Input: part model. Units: mm. Frame: model coordinates. A direction names the side the tool comes from. Give positions to 0.01 mm unless a question says otherwise; leave off trailing zeros. Loops run counter-clockwise (first coordinate to the right, second up) from the corner with the lowest first, then second, coordinate; pieces in that order, holes last. Notation, with made-up numbers: (55.25, -39.75) - (71.25, -39.75) arc R12 cw to (71.25, -19.75) - close; hole circle Ø8 at (-28.75, 45). An arc over 180 degrees is marked (long way). Answer as a JSON object with one key per item and string values.
from build123d import *

# Parameters (mm, degrees)
SKETCH1_R           = 2.54
SKETCH1_W           = 20.32
SKETCH1_H           = 25.4
BOSS_EXTRUDE1_DEPTH = 3.175


with BuildPart() as part:
    # Sketch1 → Boss-Extrude1 (new body)
    with BuildSketch(Plane(origin=(0, 0, 0), x_dir=(1, 0, 0), z_dir=(0, 1, 0))):
        with BuildLine():
            Line((-28.4999938, 15.7999938), (-28.4999938, 9.525))
            Line((-28.4999938, 9.525), (-36.1199938, 9.525))
            ThreePointArc((-36.1199938, 9.525), (-39.712096248, 8.037102448), (-41.1999938, 4.445))
            Line((-41.1999938, 4.445), (-41.1999938, -4.445))
            ThreePointArc((-41.1999938, -4.445), (-39.712096248, -8.037102448), (-36.1199938, -9.525))
            Line((-36.1199938, -9.525), (-28.4999938, -9.525))
            Line((-28.4999938, -9.525), (-28.4999938, -15.7999938))
            Line((-28.4999938, -15.7999938), (-15.7999938, -15.7999938))
            Line((-15.7999938, -15.7999938), (-15.7999938, -28.4999938))
            Line((-15.7999938, -28.4999938), (15.7999938, -28.4999938))
            Line((15.7999938, -28.4999938), (15.7999938, -15.7999938))
            Line((15.7999938, -15.7999938), (28.4999938, -15.7999938))
            Line((28.4999938, -15.7999938), (28.4999938, -9.525))
            Line((28.4999938, -9.525), (36.1199938, -9.525))
            ThreePointArc((36.1199938, -9.525), (39.712096248, -8.037102448), (41.1999938, -4.445))
            Line((41.1999938, -4.445), (41.1999938, 4.445))
            ThreePointArc((41.1999938, 4.445), (39.712096248, 8.037102448), (36.1199938, 9.525))
            Line((36.1199938, 9.525), (28.4999938, 9.525))
            Line((28.4999938, 9.525), (28.4999938, 15.7999938))
            Line((28.4999938, 15.7999938), (15.7999938, 15.7999938))
            Line((15.7999938, 15.7999938), (15.7999938, 28.4999938))
            Line((15.7999938, 28.4999938), (-15.7999938, 28.4999938))
            Line((-15.7999938, 28.4999938), (-15.7999938, 15.7999938))
            Line((-15.7999938, 15.7999938), (-28.4999938, 15.7999938))
        make_face()
        with Locations((-34.8499938, 0)):
            Circle(SKETCH1_R, mode=Mode.SUBTRACT)
        with Locations((34.8499938, 0)):
            Circle(SKETCH1_R, mode=Mode.SUBTRACT)
        Rectangle(SKETCH1_W, SKETCH1_H, mode=Mode.SUBTRACT)
    extrude(amount=BOSS_EXTRUDE1_DEPTH)


solid = part.part
Item 1: Cut plane B-B (y = 2.2). Give the number of separate pieces and of enclosed holes in the cut face, then the cut area to 3 significant figures.
Geometry check:
{"separate pieces": "1", "enclosed holes": "3", "area": "2,510 mm2"}
Item 2: Mould query, pull axis X, two halves, no side actions, for faces 5 (the face through (-28.5, 2, 13)), 6 (the face through (32.312, 1.565, -0.112)), 7 (the face through (0, 2, 28.5)), 8 (the face through (39.67, 1.57, 8.08)). Classes: released by +X, released by -X, zero draft, split by the parting line, or undercut.
Geometry check:
{"face 5": "released by -X", "face 6": "undercut", "face 7": "zero draft", "face 8": "released by +X"}
Item 3: Cut plane C-C (x = -20). Return loops of the section in (y, z) (3 decimals).
Geometry check:
{"outline": "(0, -15.8) - (3.175, -15.8) - (3.175, 15.8) - (0, 15.8) - close"}
Item 4: Contact query for flat-ended pins moving along their axis: P1, Ø1, axis at x = -30.5, y = 1, coming from the +Z side (3 decimals); P2, Ø1, axis at x = -21, y = 1, coming from the -Z side; P3, Ø1, axis at x = -21, y = 1.5, coming from the +Z side; P4, Ø4.5, axis at x = 34.85, z = 0, coming from the +Y side. Output: stop coordinate, or through.
Geometry check:
{"P1": "stops at z = 9.525", "P2": "stops at z = -15.8", "P3": "stops at z = 15.8", "P4": "passes through"}
Item 5: Access query for faces 1 (the face through (0, 2, 12.7)), 2 (the face through (28.5, 2, -13)), 3 (the face through (28.5, 2, 13)), 4 (the face through (-15.8, 2, -22)). Directions: +Z, -Z, +X, -X, +Y, -Y. A direction counts if a zero-diameter tool reaches every point of the face in a straight line with its end or side. Return the directions, or none.
Geometry check:
{"face 1": "+Y, -Y", "face 2": "-Z, +X, +Y, -Y", "face 3": "+Z, +X, +Y, -Y", "face 4": "-Z, -X, +Y, -Y"}
Item 6: Cut plane A-A (z = 0). Return loops of the section in (x, y) (3 decimals).
Geometry check:
{"outline": "(-41.2, 0) - (-37.39, 0) - (-37.39, 3.175) - (-41.2, 3.175) - close; (-32.31, 0) - (-10.16, 0) - (-10.16, 3.175) - (-32.31, 3.175) - close; (10.16, 0) - (32.31, 0) - (32.31, 3.175) - (10.16, 3.175) - close; (37.39, 0) - (41.2, 0) - (41.2, 3.175) - (37.39, 3.175) - close"}
Item 7: Material intervals for line 1 (X direction, y = 2.25, z = 0); line 2 (Z direction, x = 0, y = 2.3); line 3 (Z direction, x = 35, y = 2.05) (3 decimals), sorted ascending. Write a range as [from, to].
Geometry check:
{"line 1": "x = [-41.2, -37.39], [-32.31, -10.16], [10.16, 32.31], [37.39, 41.2]", "line 2": "z = [-28.5, -12.7], [12.7, 28.5]", "line 3": "z = [-9.525, -2.536], [2.536, 9.525]"}
